from build123d import *

# Parameters (mm, degrees)
SKIZZE1_R                       = 2.7
AUFSATZ_LINEAR_AUSTRAGEN2_DEPTH = 2.9
SKIZZE3_R                       = 1.45
AUFSATZ_LINEAR_AUSTRAGEN3_DEPTH = 12
FASE1_SIZE                      = 0.1


with BuildPart() as part:
    # Skizze1 → Aufsatz-Linear austragen2 (new body)
    with BuildSketch(Plane.XY):
        Circle(SKIZZE1_R)
    extrude(amount=AUFSATZ_LINEAR_AUSTRAGEN2_DEPTH)

    # Skizze3 → Aufsatz-Linear austragen3 (add)
    with BuildSketch(Plane.XY.offset(2.9)):
        Circle(SKIZZE3_R)
    extrude(amount=AUFSATZ_LINEAR_AUSTRAGEN3_DEPTH)

    # Fase1
    fase1_edges = [part.edges().sort_by_distance(p)[0] for p in [
        (-1.45, 0, 14.9),
    ]]
    chamfer(fase1_edges, length=FASE1_SIZE)


solid = part.part
Verification items for the finished model (mm, model axes). A direction names the side the tool comes from. Give positions to 0.01 mm unless a question says otherwise; leave off trailing zeros. Loops run counter-clockwise (first coordinate to the right, second up) from the corner with the lowest first, then second, coordinate; pieces in that order, holes last.
1) Sectioned sample at C-C, the plane z = 5.5. Enter the section's corners in (x, y).
2) Depth check by flat-ended pin: pin 1 Ø1 at (y, z) = (-1, 5) entering from -X; pin 2 Ø1.5 at (x, z) = (-1, 3) entering from +Y; pin 3 Ø1 at (x, z) = (0, 11.5) entering from +Y. Enter the tip coordinate at first touch or a pass-through.
3) Set-up check for faces 1 (the flat face through (0, 0, 14.9)), 2 (the cylindrical face through (-1.45, 0.06, 8.77)): record each of +Z, -Z, +X, -X, +Y, -Y from which the full face is reachable in a straight line by a thin tool's end or side.
4) Sectioned sample at D-D, the plane z = 1.25. Enter the section's corners in (x, y).
5) Thickness scan on line 1 along Z through (x, y) = (1.5, 2.1); line 2 along X through (y, z) = (-0.05, 14.25); line 3 along X through (y, z) = (-1, 10.25). Record the ranges inside material, lowest first.
6) Sectioned sample at A-A, the plane x = 0. Enter the section's corners in (y, z), then the cut area to 4 significant figures.
Answers:
1. outline: circle Ø2.9 at (0, 0)
2. pin 1: stops at x = -1.36
2. pin 2: stops at y = 2.69
2. pin 3: stops at y = 1.45
3. face 1: +Z, +X, -X, +Y, -Y
3. face 2: +Z
4. outline: circle Ø5.4 at (0, 0)
5. line 1: z = 0 to 2.9
5. line 2: x = -1.45 to 1.45
5. line 3: x = -1.05 to 1.05
6. outline: (-2.7, 0) - (2.7, 0) - (2.7, 2.9) - (1.45, 2.9) - (1.45, 14.8) - (1.35, 14.9) - (-1.35, 14.9) - (-1.45, 14.8) - (-1.45, 2.9) - (-2.7, 2.9) - close
6. area: 50.45 mm2
